```python
from build123d import *

# Parameters (mm, degrees)
EXTRUDE1_DEPTH     = 5.08
SKETCH4_R          = 10.674627582
EXTRUDE2_DEPTH     = 2.54
SKETCH6_R          = 3.225
CUT_EXTRUDE1_DEPTH = 29.049397538
EXTRUDE3_DEPTH     = 2.54


with BuildPart() as part:
    # Sketch3 → Extrude1 (new, symmetric)
    with BuildSketch(Plane.XY):
        with BuildLine():
            Line((17.977749936, -9.697339402), (0, -9.697339402))
            Line((0, -9.697339402), (0, -0.708464433))
            ThreePointArc((0, -0.708464433), (8.988874968, 8.280410535), (17.977749936, -0.708464433))
            Line((17.977749936, -0.708464433), (17.977749936, -9.697339402))
        make_face()
    extrude(amount=EXTRUDE1_DEPTH, both=True)

    # Sketch4 → Extrude2 (add)
    with BuildSketch(Plane.XZ.offset(9.697339402)):
        with Locations((9.043585733, 0)):
            Circle(SKETCH4_R)
    extrude(amount=EXTRUDE2_DEPTH)

    # Sketch6 → Cut-Extrude1 (cut, through all)
    with BuildSketch(Plane.XY.offset(5.08)):
        with Locations((8.988874968, -0.708464433)):
            Circle(SKETCH6_R)
    extrude(amount=-CUT_EXTRUDE1_DEPTH, mode=Mode.SUBTRACT)

    # Sketch8 → Extrude3 (cut)
    with BuildSketch(Plane.XY.offset(5.08)):
        with BuildLine():
            Line((0.254, -9.697339402), (0, -9.697339402))
            Line((0, -9.697339402), (0, -0.708464433))
            ThreePointArc((0, -0.708464433), (8.988874968, 8.280410535), (17.977749936, -0.708464433))
            Line((17.977749936, -0.708464433), (17.977749936, -9.697339402))
            Line((17.977749936, -9.697339402), (17.723749936, -9.697339402))
            Line((17.723749936, -9.697339402), (17.723749936, -0.708464433))
            ThreePointArc((17.723749936, -0.708464433), (8.988874968, 8.026410535), (0.254, -0.708464433))
            Line((0.254, -0.708464433), (0.254, -9.697339402))
        make_face()
    extrude3 = extrude(amount=-EXTRUDE3_DEPTH, mode=Mode.SUBTRACT)

    # Mirror1: Extrude3 across plane
    add(extrude3.mirror(Plane.XY), mode=Mode.SUBTRACT)


solid = part.part
```
Can you work these out from the model? Positions are in its coordinate system, mm. A direction names the side the tool comes from. Coordinates: 2 decimals unless noted, no trailing zeros. Loops run counter-clockwise (first coordinate to the right, second up) from the corner with the lowest first, then second, coordinate; pieces in that order, holes last.
Item 1: If we mould it in two halves opening along Y, with no side actions, what happens to faces 1 (the face through (9.181, 8.024, -3.828)), 2 (the face through (6.73, -10.95, -10.42)), 3 (the face through (11.97, -1.94, 0.07))? For each: released by +Y, released by -Y, zero draft, split by the parting line, or undercut.
Answers below:
face 1: released by +Y
face 2: zero draft
face 3: undercut
Item 2: Suppose I cut it at C-C (x = 1.5). Please give me the cut outline in (y, z), then the cut area to 3 significant figures.
Answers below:
outline: (-12.24, -7.55) - (-9.7, -7.55) - (-9.7, -5.08) - (3.79, -5.08) - (3.79, -2.54) - (4.26, -2.54) - (4.26, 2.54) - (3.79, 2.54) - (3.79, 5.08) - (-9.7, 5.08) - (-9.7, 7.55) - (-12.24, 7.55) - close
area: 178 mm2
Item 3: Suppose I cut it at A-A (z = 0). Please give me the cut outline in (x, y) (3 decimals), then the cut area to 3 significant figures.
Answers below:
outline: (-1.631, -12.237) - (19.718, -12.237) - (19.718, -9.697) - (17.978, -9.697) - (17.978, -0.708) arc R8.989 ccw to (0, -0.708) - (0, -9.697) - (-1.631, -9.697) - close; hole circle Ø6.45 at (8.989, -0.708)
area: 310 mm2
Item 4: Suppose I cut it at B-B (y = 2). Please give me the cut outline in (x, z), then the cut area to 3 significant figures.
Answers below:
outline: (0.42, -2.54) - (0.68, -2.54) - (0.68, -5.08) - (7.24, -5.08) - (7.24, 5.08) - (0.68, 5.08) - (0.68, 2.54) - (0.42, 2.54) - close; (10.74, -5.08) - (17.29, -5.08) - (17.29, -2.54) - (17.56, -2.54) - (17.56, 2.54) - (17.29, 2.54) - (17.29, 5.08) - (10.74, 5.08) - close
area: 136 mm2
Item 5: I'm going to push flat-ended pins straight in: pin 1 (0.8 mm diameter, centred on y = -6, z = -3.5, fed in from +X); pin 2 (5.5 mm diameter, centred on x = 6.5, y = -3, fed in from +Z); pin 3 (6 mm diameter, centred on x = 1.5, y = -9.5, fed in from +Z); pin 4 (2 mm diameter, centred on x = 10.5, y = -1, fed in from -Z). Where does each tip first touch, or does it pass through?
Answers below:
pin 1: stops at x = 17.72
pin 2: stops at z = 5.08
pin 3: stops at z = 9.66
pin 4: passes through
Item 6: Which directions (+Z, -Z, +X, -X, +Y, -Y) give clear straight access to the entire face, cutting with the end or side of a thin tool? Please do faces 4 (the face through (9, -5, -5.08)), 5 (the face through (0.254, -5, -4)), 6 (the face through (17.724, -5, -4)), 7 (the face through (9, -5, 5.08)).
Answers below:
face 4: -Z, +X, -X, +Y
face 5: -Z, -X, +Y
face 6: -Z, +X, +Y
face 7: +Z, +X, -X, +Y
Item 7: Suppose I cut it at D-D (y = -11). Please give me the cut outline in (x, z), then the cut area to 3 significant figures.
Answers below:
outline: circle Ø21.35 at (9.04, 0)
area: 358 mm2
Item 8: Please list where these lines run through material, in increasing order: L1, parallel to Z at x = 10.75, y = 3.5; L2, parallel to X at y = -8, z = -2; L3, parallel to Y at x = 11.75, z = 6.5.
Answers below:
L1: z = -5.08 to 5.08
L2: x = 0 to 17.98
L3: y = -12.24 to -9.7
